from build123d import *

# Parameters (mm, degrees)
F1_DEPTH = 25.4
F2_R     = 5.08


with BuildPart() as f1:
    # F0 (on Front) → F1 (new body)
    with BuildSketch(Plane.XZ):
        with BuildLine():
            Line((5.08, 43.18), (-5.08, 43.18))
            ThreePointArc((-5.08, 43.18), (-26.632615, 34.252615), (-35.56, 12.7))
            Line((-35.56, 12.7), (-35.56, -12.7))
            ThreePointArc((-35.56, -12.7), (-26.632615, -34.252615), (-5.08, -43.18))
            Line((-5.08, -43.18), (5.08, -43.18))
            ThreePointArc((5.08, -43.18), (26.632615, -34.252615), (35.56, -12.7))
            Line((35.56, -12.7), (35.56, 0))
            Line((35.56, 0), (35.56, 2.54))
            Line((35.56, 2.54), (0, 2.54))
            Line((0, 2.54), (0, 0))
            Line((0, 0), (0, -12.7))
            Line((0, -12.7), (0, -15.24))
            Line((0, -15.24), (16.224205, -15.24))
            ThreePointArc((16.224205, -15.24), (12.207857, -21.635242), (5.08, -24.13))
            Line((5.08, -24.13), (-5.08, -24.13))
            ThreePointArc((-5.08, -24.13), (-13.162231, -20.782231), (-16.51, -12.7))
            Line((-16.51, -12.7), (-16.51, 12.7))
            ThreePointArc((-16.51, 12.7), (-13.162231, 20.782231), (-5.08, 24.13))
            Line((-5.08, 24.13), (5.08, 24.13))
            ThreePointArc((5.08, 24.13), (13.162231, 20.782231), (16.51, 12.7))
            Line((16.51, 12.7), (35.56, 12.7))
            ThreePointArc((35.56, 12.7), (26.632615, 34.252615), (5.08, 43.18))
        make_face()
    extrude(amount=F1_DEPTH)

    # F2
    f2_edges = [f1.edges().sort_by_distance(p)[0] for p in [
        (26.632615, -25.4, 34.252615),
        (-13.162231, -25.4, -20.782231),
        (8.112102, -25.4, -15.24),
        (0, -25.4, -6.35),
        (17.78, -25.4, 2.54),
        (26.035, -25.4, 12.7),
    ]]
    fillet(f2_edges, radius=F2_R)


solid = f1.part
Check sheet for the modelled part. Datum: model origin and axes. Units: mm. A direction names the side the tool comes from. Round coordinates to 2 decimals unless told otherwise and drop trailing zeros. Loops run counter-clockwise (first coordinate to the right, second up) from the corner with the lowest first, then second, coordinate; pieces in that order, holes last.
1. Gauge pin test, flat ends, axial feed: pin 1 Ø8 at (x, z) = (14, 6) entering from -Y; pin 2 Ø3 at (x, y) = (-10.5, -13.5) entering from +Z; pin 3 Ø8 at (x, y) = (9.5, -11.5) entering from -Z. Record the tip position at first contact, or that the pin passes through.
2. Set-up check for faces 4 (the flat face through (7, 0, 1)), 5 (the cylindrical face through (0.89, -23.19, -6.47)), 6 (the flat face through (0, -10, 24.13)): record each of +Z, -Z, +X, -X, +Y, -Y from which the full face is reachable in a straight line by a thin tool's end or side.
3. Sectioned sample at A-A on y = -19. Record the boundary of the cut face in (x, z), and give its area (3 significant figures).
4. Scan lines: probe 1 along X at (y, z) = (-3.5, -7); probe 2 along Z at (x, y) = (15, -11.75); probe 3 along Z at (x, y) = (-4, -9). Record each from-to range of solid material in increasing order.
5. Mould release check, pull along X, two halves, no side actions. Record for faces 1 (the flat face through (0, -10, -6)), 2 (the flat face through (26, -10, 12.7)), 3 (the flat face through (-35.56, -10, 0)): released by +X, released by -X, zero draft, split by the parting line, or undercut.
6. Sectioned sample at B-B on x = 6. Give the number of separate pieces and of enclosed holes in the cut face, and give its area (3 significant figures).
Recorded:
1. pin 1: stops at y = -22.6
1. pin 2: stops at z = 42.93
1. pin 3: stops at z = -43.18
2. face 4: +Z, -Z, +X, -X, +Y
2. face 5: -Y
2. face 6: +Y, -Y
3. outline: (-35.56, -12.7) arc R30.48 ccw to (-5.08, -43.18) - (5.08, -43.18) arc R30.48 ccw to (35.56, -12.7) - (35.56, 2.54) - (0, 2.54) - (0, -15.24) - (16.22, -15.24) arc R11.43 cw to (5.08, -24.13) - (-5.08, -24.13) arc R11.43 cw to (-16.51, -12.7) - (-16.51, 12.7) arc R11.43 cw to (-5.08, 24.13) - (5.08, 24.13) arc R11.43 cw to (16.51, 12.7) - (35.56, 12.7) arc R30.48 ccw to (5.08, 43.18) - (-5.08, 43.18) arc R30.48 ccw to (-35.56, 12.7) - close
3. area: 3,960 mm2
4. probe 1: x = -35.56 to -16.51, 0 to 35.56
4. probe 2: z = -41.52 to -18.38, -15.24 to 2.54, 18.38 to 41.52
4. probe 3: z = -43.18 to -24.13, 24.13 to 43.18
5. face 1: undercut
5. face 2: zero draft
5. face 3: released by -X
6. separate pieces: 3
6. enclosed holes: 0
6. area: 1,390 mm2
